The listing builds one solid part. Answer for the finished solid, in the listing's coordinates (mm). A direction names the side the tool comes from. Give positions to 0.01 mm unless a question says otherwise; leave off trailing zeros. Order: outer loops, then holes, each group sorted by start corner. A loop starts at its lowest first (then second) coordinate and runs counter-clockwise, first axis right, second up.
```python
from build123d import *

# Parameters (mm, degrees)
SKETCH1_R           = 1.28
SKETCH1_R_2         = 2.38125
SKETCH1_R_3         = 1.53
BASE_DEPTH          = 6
ALL_CUTS_DEPTH      = 76.612498967
ALL_CUTS_DEPTH_BACK = 76.612498967
SKETCH2_W           = 5
SKETCH2_H           = 40
SKETCH2_W_2         = 6
SKETCH2_H_2         = 20
SKETCH2_H_3         = 52.5
SKETCH2_W_3         = 8
SKETCH3_W           = 16
SKETCH3_H           = 24
SKETCH3_W_2         = 8
SKETCH3_H_2         = 20
BOSS_EXTRUDE1_DEPTH = 15
SKETCH4_R           = 2.38125
CUT_EXTRUDE1_DEPTH  = 78.053552806
FILLET1_R           = 2.5
FILLET2_R           = 8
FILLET3_R           = 8
BOSS_EXTRUDE2_DEPTH = 1


with BuildPart() as part:
    # Sketch1 → BASE (new, symmetric)
    with BuildSketch(Plane(origin=(0, 0, 0), x_dir=(0, 0, -1), z_dir=(1, 0, 0))):
        with BuildLine():
            Line((-67.5, 7.5), (67.5, 7.5))
            ThreePointArc((67.5, 7.5), (75, 0), (67.5, -7.5))
            Line((67.5, -7.5), (-67.5, -7.5))
            ThreePointArc((-67.5, -7.5), (-75, 0), (-67.5, 7.5))
        make_face()
        with Locations((-67.5, 0)):
            Circle(SKETCH1_R, mode=Mode.SUBTRACT)
        Circle(SKETCH1_R_2, mode=Mode.SUBTRACT)
        with Locations((67.5, 0)):
            Circle(SKETCH1_R_3, mode=Mode.SUBTRACT)
    extrude(amount=BASE_DEPTH, both=True)

    # Sketch2 → All_Cuts (cut, two sides: drawn at the far end of the back side and taken through both)
    with BuildSketch(Plane(origin=(0, 0, 0), x_dir=(1, 0, 0), z_dir=(0, 1, 0)).offset(-ALL_CUTS_DEPTH_BACK)):
        with Locations((0, -75)):
            Rectangle(SKETCH2_W, SKETCH2_H)
        with Locations((-6, -30)):
            Rectangle(SKETCH2_W_2, SKETCH2_H_2)
        with Locations((6, -30)):
            Rectangle(SKETCH2_W_2, SKETCH2_H_2)
        with Locations((6, 48.75)):
            Rectangle(SKETCH2_W_2, SKETCH2_H_3)
        with Locations((-6, 48.75)):
            Rectangle(SKETCH2_W_2, SKETCH2_H_3)
        Rectangle(SKETCH2_W_3, SKETCH2_H_2)
    extrude(amount=ALL_CUTS_DEPTH + ALL_CUTS_DEPTH_BACK, mode=Mode.SUBTRACT)

    # Sketch3 → Boss-Extrude1 (add, through all)
    with BuildSketch(Plane.XZ.offset(7.5)):
        Rectangle(SKETCH3_W, SKETCH3_H)
        Rectangle(SKETCH3_W_2, SKETCH3_H_2, mode=Mode.SUBTRACT)
    extrude(amount=-BOSS_EXTRUDE1_DEPTH)

    # Sketch4 → Cut-Extrude1 (cut, through all)
    with BuildSketch(Plane.ZY.offset(8)):
        Circle(SKETCH4_R)
    extrude(amount=-CUT_EXTRUDE1_DEPTH, mode=Mode.SUBTRACT)

    # Fillet1
    fillet1_edges = [part.edges().sort_by_distance(p)[0] for p in [
        (3, 0, 20),
        (3, 0, 40),
        (-3, 0, 40),
        (-3, 0, 20),
        (3, 0, -22.5),
        (-3, 0, -22.5),
    ]]
    fillet(fillet1_edges, radius=FILLET1_R)

    # Fillet2
    # the kernel refuses this fillet: 8 mm, written as the material it adds along each edge
    with BuildSketch(Plane(origin=(-6, -7.5, -12), x_dir=(0, 0, -1), z_dir=(0, 1, 0))) as fillet2_piece_1:
        with BuildLine():
            CenterArc((5.291502622, 8), FILLET2_R, 228.590377891, 41.409622109)
            Line((0, 2), (-0.105830052, 1.88))
            ThreePointArc((-0.105830052, 1.88), (-0.16, 1), (-0.16, 0))
            Line((-0.16, 0), (0, -0.16))
            Line((0, -0.16), (5.291502622, -0.16))
            Line((5.291502622, -0.16), (5.291502622, 0))
        make_face()
    extrude(amount=15)
    with BuildSketch(Plane(origin=(6, -7.5, -12), x_dir=(1, 0, 0), z_dir=(0, 1, 0))) as fillet2_piece_2:
        with BuildLine():
            CenterArc((8, 5.291502622), FILLET2_R, 180, 41.409622109)
            Line((0, 5.291502622), (-0.16, 5.291502622))
            Line((-0.16, 5.291502622), (-0.16, 0))
            Line((-0.16, 0), (0, -0.16))
            ThreePointArc((0, -0.16), (1, -0.16), (1.88, -0.105830052))
            Line((1.88, -0.105830052), (2, 0))
        make_face()
    extrude(amount=15)
    with BuildSketch(Plane(origin=(6, 7.5, 12), x_dir=(0, 0, 1), z_dir=(0, -1, 0))) as fillet2_piece_3:
        with BuildLine():
            CenterArc((5.291502622, -8), FILLET2_R, 90, 41.409622109)
            Line((0, -2), (-0.105830052, -1.88))
            ThreePointArc((-0.105830052, -1.88), (-0.16, -1), (-0.16, 0))
            Line((-0.16, 0), (0, 0.16))
            Line((0, 0.16), (5.291502622, 0.16))
            Line((5.291502622, 0.16), (5.291502622, 0))
        make_face()
    extrude(amount=15)
    with BuildSketch(Plane(origin=(-6, 7.5, 12), x_dir=(-1, 0, 0), z_dir=(0, -1, 0))) as fillet2_piece_4:
        with BuildLine():
            CenterArc((8, -5.291502622), FILLET2_R, 138.590377891, 41.409622109)
            Line((0, -5.291502622), (-0.16, -5.291502622))
            Line((-0.16, -5.291502622), (-0.16, 0))
            Line((-0.16, 0), (0, 0.16))
            ThreePointArc((0, 0.16), (1, 0.16), (1.88, 0.105830052))
            Line((1.88, 0.105830052), (2, 0))
        make_face()
    extrude(amount=15)

    # Fillet3
    fillet3_edges = [part.edges().sort_by_distance(p)[0] for p in [
        (8, 0, -12),
        (-8, 0, -12),
        (-6, 0, 20),
        (6, 0, 20),
        (-6, 0, -22.5),
        (6, 0, -22.5),
        (6, 0, 40),
        (-6, 0, 40),
    ]]
    fillet(fillet3_edges, radius=FILLET3_R)

    # Sketch5 → Boss-Extrude2 (add)
    # profile 1 of 2: a face of its own
    with BuildSketch(Plane(origin=(0, 7.5, 0), x_dir=(1, 0, 0), z_dir=(0, 1, 0))):
        Polygon((-1.663472098, -13.613490945), (-1.082899181, -13.613490945), (-1.082899181, -16.753490945), (-1.364694053, -16.753490945), (-1.364694053, -13.935542228), (-1.847770976, -13.935542228), align=None)
    # profile 2 of 2: a face of its own
    with BuildSketch(Plane(origin=(0, 7.5, 0), x_dir=(1, 0, 0), z_dir=(0, 1, 0))):
        with BuildLine():
            Line((1.533767485, -13.532978125), (1.750774697, -13.703438862))
            Line((1.750774697, -13.703438862), (0.921115242, -14.972144792))
            add(Edge.make_bspline(
                [(0.921115242, -14.972144792), (0.976352576, -14.963340357), (1.084099242, -14.946166311), (1.193161219, -14.943333183), (1.246311556, -14.941952484)],
                knots=[0, 0, 0, 0, 1.025318673, 2, 2, 2, 2], degree=3))
            add(Edge.make_bspline(
                [(1.246311556, -14.941952484), (1.278225167, -14.942810253), (1.341046161, -14.944498745), (1.433278549, -14.957492828), (1.521906337, -14.977970214), (1.606562183, -15.007820181), (1.687549944, -15.045950865), (1.76533438, -15.091650308), (1.838453326, -15.147278262), (1.907848384, -15.209418822), (1.970852123, -15.278244917), (2.026632927, -15.351273544), (2.07348782, -15.42842862), (2.111503281, -15.509671066), (2.141023658, -15.594875647), (2.162544002, -15.68393335), (2.175265123, -15.776905584), (2.176992563, -15.840134576), (2.17787005, -15.872252965)],
                knots=[0, 0, 0, 0, 1.04369286, 2.054478336, 3.041073146, 4.015093852, 4.984733326, 5.965804835, 6.960378782, 7.985147595, 9.009457201, 10.008161701, 10.986880575, 11.956520048, 12.937015923, 13.931873656, 14.949455224, 16, 16, 16, 16], degree=3))
            add(Edge.make_bspline(
                [(2.17787005, -15.872252965), (2.176593321, -15.916194756), (2.174081022, -16.002661803), (2.149047331, -16.128599762), (2.110147535, -16.248576933), (2.054544838, -16.360677779), (1.985480643, -16.464748655), (1.901259031, -16.556961901), (1.804866873, -16.639203021), (1.69587586, -16.707974959), (1.578580744, -16.764138839), (1.45535638, -16.804479085), (1.327399455, -16.829315112), (1.240551892, -16.832428738), (1.19662005, -16.834003766)],
                knots=[0, 0, 0, 0, 1.031375318, 2.029502543, 3.004789286, 3.987476834, 4.960371455, 5.9300674, 6.912260825, 7.929083631, 8.949397511, 9.960523116, 10.96833055, 12, 12, 12, 12], degree=3))
            add(Edge.make_bspline(
                [(1.19662005, -16.834003766), (1.154367581, -16.832632747), (1.070672839, -16.829916999), (0.947555417, -16.8057247), (0.829255453, -16.766513185), (0.71660178, -16.712492375), (0.612245573, -16.644257589), (0.518883831, -16.562113144), (0.436982067, -16.467814938), (0.368821979, -16.361377598), (0.314761288, -16.247000893), (0.274219469, -16.127737273), (0.250538268, -16.00402129), (0.247229106, -15.920155353), (0.245562357, -15.877914022)],
                knots=[0, 0, 0, 0, 1.012016664, 2.004627821, 2.994792927, 3.992885782, 4.990978636, 5.973936114, 6.964471063, 7.975201453, 8.993600317, 9.990122807, 10.98767138, 12, 12, 12, 12], degree=3))
            add(Edge.make_bspline(
                [(0.245562357, -15.877914022), (0.246622282, -15.845576882), (0.248786446, -15.77955062), (0.263897374, -15.679551463), (0.288178361, -15.57723135), (0.315370982, -15.490429016), (0.344102529, -15.419320108), (0.368013665, -15.361989548), (0.397775479, -15.302992471), (0.429510455, -15.240305837), (0.466075189, -15.175545192), (0.505832657, -15.107628186), (0.549882058, -15.037634959), (0.580761861, -14.990136453), (0.596547934, -14.965854728)],
                knots=[0, 0, 0, 0, 1.173818275, 2.396712641, 3.66331629, 4.989737886, 5.693666774, 6.447286557, 7.243889047, 8.091586357, 8.998013824, 9.943181721, 10.948533338, 12, 12, 12, 12], degree=3))
            Line((0.596547934, -14.965854728), (1.533767485, -13.532978125))
        make_face()
        with BuildLine():
            add(Edge.make_bspline(
                [(1.187184953, -15.264003766), (1.163265111, -15.264701782), (1.11654271, -15.266065211), (1.047994344, -15.273982723), (0.983119027, -15.288892399), (0.921057255, -15.307881622), (0.862969316, -15.333991224), (0.808433043, -15.365706838), (0.757237539, -15.403046981), (0.709919038, -15.445482655), (0.667017969, -15.491943919), (0.630072611, -15.541708005), (0.598203944, -15.593575604), (0.572292826, -15.64798009), (0.552116016, -15.704900664), (0.537521071, -15.764075533), (0.529398562, -15.82590151), (0.528047257, -15.867827242), (0.527357229, -15.889236138)],
                knots=[0, 0, 0, 0, 1.129588631, 2.206414736, 3.251139165, 4.268635594, 5.265702196, 6.250456724, 7.242448911, 8.251968645, 9.246821453, 10.222880186, 11.173611482, 12.116736599, 13.062300278, 14.020270554, 14.989073742, 16, 16, 16, 16], degree=3))
            add(Edge.make_bspline(
                [(0.527357229, -15.889236138), (0.527919165, -15.910453548), (0.529021037, -15.952057732), (0.539026261, -16.013367738), (0.554309164, -16.072368256), (0.577043119, -16.128755119), (0.604160956, -16.183387816), (0.639961732, -16.234287472), (0.679630506, -16.284545478), (0.727048035, -16.330301084), (0.777936995, -16.372876455), (0.83230493, -16.410090168), (0.888968437, -16.441926335), (0.948692513, -16.466876863), (1.010629806, -16.487353509), (1.07529636, -16.50176295), (1.142737151, -16.509909479), (1.188421404, -16.511262544), (1.211716203, -16.511952484)],
                knots=[0, 0, 0, 0, 0.989467248, 1.94019797, 2.891935182, 3.827694429, 4.772920941, 5.730924762, 6.725747692, 7.756678648, 8.79901574, 9.819492441, 10.826891316, 11.826466727, 12.835195252, 13.867842842, 14.912794438, 16, 16, 16, 16], degree=3))
            add(Edge.make_bspline(
                [(1.211716203, -16.511952484), (1.235010965, -16.51126249), (1.280695143, -16.509909319), (1.348136476, -16.501763559), (1.412801025, -16.487351275), (1.474745607, -16.466884961), (1.534442776, -16.441896294), (1.591056726, -16.410288229), (1.644910502, -16.372647597), (1.695832868, -16.330373842), (1.74305303, -16.284285055), (1.783673217, -16.234736104), (1.818377604, -16.182976438), (1.84657856, -16.128970331), (1.869062119, -16.072334162), (1.884422521, -16.013376872), (1.894407083, -15.95205534), (1.895511794, -15.910452741), (1.896075178, -15.889236138)],
                knots=[0, 0, 0, 0, 1.087397944, 2.132534446, 3.165364764, 4.174271784, 5.174024072, 6.181601208, 7.194203697, 8.236725232, 9.267838612, 10.269026844, 11.221737037, 12.171628256, 13.107553087, 14.05945871, 15.010357665, 16, 16, 16, 16], degree=3))
            add(Edge.make_bspline(
                [(1.896075178, -15.889236138), (1.895581486, -15.867799312), (1.894612531, -15.825725795), (1.88365308, -15.764103189), (1.86845335, -15.704600004), (1.845501717, -15.64759021), (1.815683788, -15.593298778), (1.779364389, -15.541451456), (1.737348883, -15.491650744), (1.688815661, -15.445391539), (1.635982709, -15.403093875), (1.579807583, -15.365755187), (1.521037573, -15.334243065), (1.459732264, -15.307950408), (1.395189221, -15.288976308), (1.32845046, -15.27403597), (1.258662396, -15.266085474), (1.211314239, -15.264706507), (1.187184953, -15.264003766)],
                knots=[0, 0, 0, 0, 0.978206639, 1.919901502, 2.851605144, 3.780102724, 4.718870031, 5.675451981, 6.667674623, 7.690630536, 8.733308323, 9.756129687, 10.767539656, 11.776269907, 12.797430371, 13.836405707, 14.897401972, 16, 16, 16, 16], degree=3))
        make_face(mode=Mode.SUBTRACT)
    extrude(amount=BOSS_EXTRUDE2_DEPTH)


solid = part.part
```
1) Find section A-A (z = 0). Write down the section's boundary in (x, y).
Geometry says:
outline: (-8, -7.5) - (-4, -7.5) - (-4, -2.38) - (-8, -2.38) - close; (-8, 2.38) - (-4, 2.38) - (-4, 7.5) - (-8, 7.5) - close; (4, -7.5) - (8, -7.5) - (8, -2.38) - (4, -2.38) - close; (4, 2.38) - (8, 2.38) - (8, 7.5) - (4, 7.5) - close
2) Given P1, Ø4.5, axis at y = 2.5, z = 60, coming from the +X side; P2, Ø1.5, axis at x = 3.5, y = -3, coming from the +Z side; P3, Ø8, axis at y = -3.5, z = 17, coming from the +X side, each flat-ended and moving along its own axis, determine where each tip first touches the part or whether it passes through.
Geometry says:
P1: stops at x = 6
P2: stops at z = 74.65
P3: stops at x = 7.25
3) A tool of negligible diameter and unlimited length cuts with its end or side. For faces 1 (the flat face through (0, 0, 55)), 2 (the flat face through (6, 0, 60)), 3 (the flat face through (0, 0, -10)), 4 (the flat face through (3, 0, 30)), from which of +Z, -Z, +X, -X, +Y, -Y can it reach the whole face along a straight path? Write none if from no direction.
Geometry says:
face 1: +Z, +Y, -Y
face 2: +Z, +X, +Y, -Y
face 3: +Y, -Y
face 4: +X, +Y, -Y
4) Find section C-C (z = -16). Write down the section's boundary in (x, y), then the cut area to 3 significant figures.
Geometry says:
outline: (-6.1, -7.5) - (6.1, -7.5) - (6.1, 7.5) - (-6.1, 7.5) - close
area: 183 mm2
5) For a pull along X with two mould halves and no side action, classify faces 5 (the flat face through (-8, 0, 3)), 6 (the flat face through (-4, -2, 2)), 7 (the cylindrical face through (4.23, 0.06, 68.78)) as +X half, -X half, draft (parallel to the pull), parting line (faces both ways), or undercut.
Geometry says:
face 5: -X half
face 6: undercut
face 7: draft
6) Straight lines are drawn through the part: probe 1 along Z at (x, y) = (0.75, 0); probe 2 along Y at (x, z) = (-3.8, 67.5); probe 3 along Z at (x, y) = (-3.5, -2.5). For each, find the intervals that lie inside material, in ascending order.
Geometry says:
probe 1: z = -75 to -69.03, -65.97 to -10, 10 to 55
probe 2: y = -7.5 to -1.28, 1.28 to 7.5
probe 3: z = -23.5 to -10, 10 to 21, 39 to 74.57
7) Find section B-B (y = 0). Count the separate pieces of the cut face and the enclosed holes in it, then the cut area to 3 significant figures.
Geometry says:
separate pieces: 5
enclosed holes: 0
area: 1,130 mm2
